```python
from build123d import *

# Parameters (mm, degrees)
SKETCH2_R           = 7.9375
BOSS_EXTRUDE1_DEPTH = 6.35
SKETCH3_W           = 1.27
SKETCH3_H           = 6.477
CUT_EXTRUDE1_DEPTH  = 7.35


with BuildPart() as part:
    # Sketch2 → Boss-Extrude1 (new body)
    with BuildSketch(Plane.XY):
        Polygon((0, 0), (63.5, 0), (63.5, 158.877), (0, 158.877), (0, 151.2062), (11.0998, 151.2062), (11.0998, 121.8438), (0, 121.8438), align=None)
        with Locations((31.75, 108.077)):
            Circle(SKETCH2_R, mode=Mode.SUBTRACT)
    extrude(amount=BOSS_EXTRUDE1_DEPTH)

    # Sketch3 → Cut-Extrude1 (cut, through all)
    with BuildSketch(Plane.XY.offset(6.35)):
        with Locations((0.635, 3.2385)):
            Rectangle(SKETCH3_W, SKETCH3_H)
        with Locations((62.865, 3.2385)):
            Rectangle(SKETCH3_W, SKETCH3_H)
    extrude(amount=-CUT_EXTRUDE1_DEPTH, mode=Mode.SUBTRACT)


solid = part.part
```
Could you check a few things on this model? Use its own coordinates, in mm. A direction names the side the tool comes from. Round coordinates to 2 decimals unless told otherwise and drop trailing zeros. Loops run counter-clockwise (first coordinate to the right, second up) from the corner with the lowest first, then second, coordinate; pieces in that order, holes last. Notation, with made-up numbers: (-25.5, 76.25) - (-18.5, 76.25) arc R19 ccw to (-18.5, 83.25) - close; hole circle Ø1 at (11, 65). An arc over 180 degrees is marked (long way). Use CSV: the item, a comma, the result in double quotes.
Item 1: For faces 1 (the flat face through (62.23, 3, 3)), 2 (the flat face through (5, 151.206, 3)), 3 (the flat face through (1.27, 3, 3)), which set-ups out of +Z, -Z, +X, -X, +Y, -Y let a thin tool reach every point of the face, with its end or its side?
Here are the results:
face 1,"+Z, -Z, +X, -Y"
face 2,"+Z, -Z, -X"
face 3,"+Z, -Z, -X, -Y"
Item 2: If we section it at C-C on y = 137: List the corners of the cut face in (x, z) for me.
Here are the results:
outline,"(11.1, 0) - (63.5, 0) - (63.5, 6.35) - (11.1, 6.35) - close"
Item 3: Will these pins go through, and if not, where does the flat tip stop? pin 1 (1 mm diameter, centred on x = 0.5, z = 4, fed in from -Y); pin 2 (1.9 mm diameter, centred on y = 136, z = 3.5, fed in from -X).
Here are the results:
pin 1,"stops at y = 6.48"
pin 2,"stops at x = 11.1"
Item 4: If we section it at A-A on x = 31.75: List the corners of the cut face in (y, z) for me, then the cut area to 3 significant figures.
Here are the results:
outline,"(0, 0) - (100.14, 0) - (100.14, 6.35) - (0, 6.35) - close; (116.01, 0) - (158.88, 0) - (158.88, 6.35) - (116.01, 6.35) - close"
area,"908 mm²"
Item 5: I need wall thicknesses on L1, parallel to Y at x = 31.75, z = 2; L2, parallel to Y at x = 10, z = 5.5; L3, parallel to X at y = 134, z = 6.25. Which ranges of each line are inside material? Lowest first, please. Write a range as [from, to].
Here are the results:
L1,"y = [0, 100.14], [116.01, 158.88]"
L2,"y = [0, 121.84], [151.21, 158.88]"
L3,"x = [11.1, 63.5]"
Item 6: If we mould it in two halves opening along Y, with no side actions, what happens to faces 4 (the flat face through (63.5, 82, 3)), 5 (the flat face through (6, 121.844, 3)), 6 (the flat face through (31, 0, 3)), 7 (the cylindrical face through (30.03, 100.33, 3.13))? For each: pulls with the +Y half, pulls with the -Y half, needs draft (parallel to the pull), parting line crosses it, or undercut.
Here are the results:
face 4,"needs draft"
face 5,"undercut"
face 6,"pulls with the -Y half"
face 7,"undercut"
